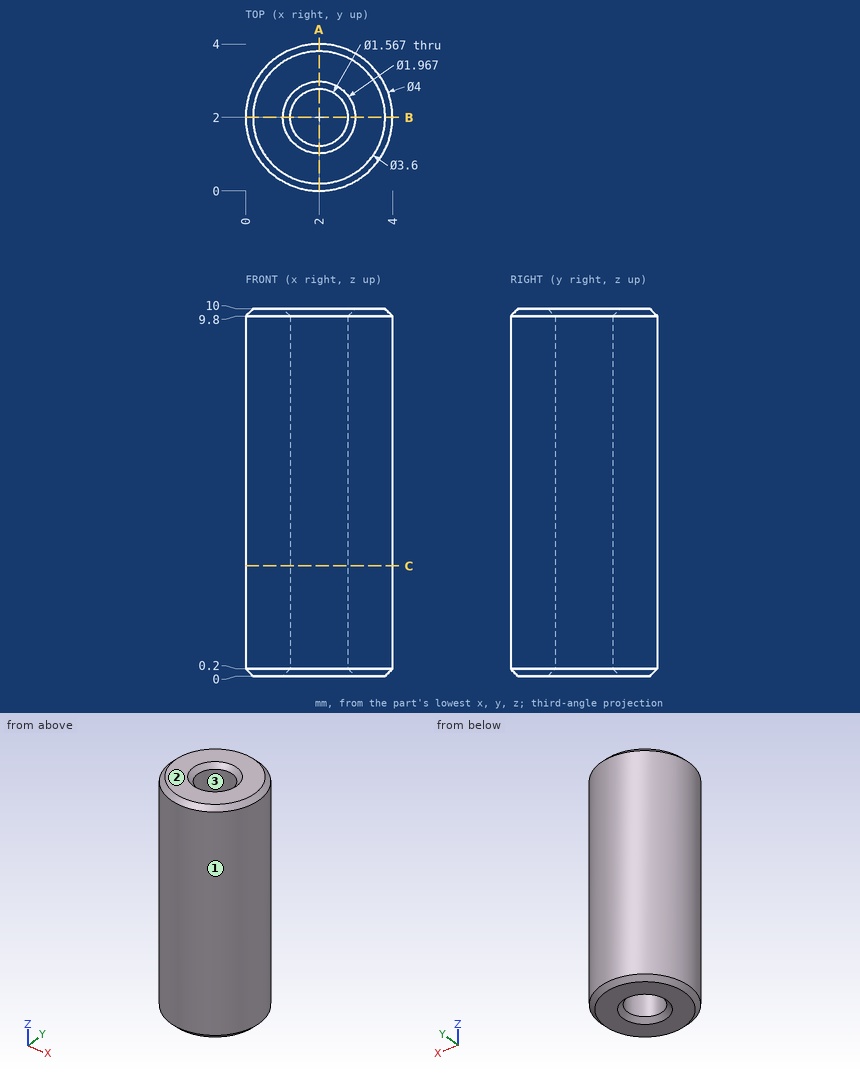
Check sheet for the drawn part. Datum: minimum x, y, z corner. Units: mm. Round coordinates to 2 decimals unless told otherwise and drop trailing zeros. Loops run counter-clockwise (first coordinate to the right, second up) from the corner with the lowest first, then second, coordinate; pieces in that order, holes last. Notation, with made-up numbers: (-36.5, -3.5) -> (8.5, -3.5) arc R11 ccw to (8.5, 0.5) -> close; hole circle Ø6 at (63.25, -30.5). An arc over 180 degrees is marked (long way). Put each result on its own line as item: value. Start each with the question number.
1. Section check C-C (z = 3). Enter the section's corners in (x, y).
2. Draft check along Y on the marked faces 1, 2 and 3. Enter one of: +Y half, -Y half, draft (parallel to the pull), parting line (faces both ways), or undercut.
3. Section check A-A (x = 2). Enter the section's corners in (y, z).
4. Gauge pin test, flat ends, axial feed: pin 1 (2 mm diameter, centred on x = 1, z = 2, fed in from -Y); pin 2 (1 mm diameter, centred on y = 1, z = 3, fed in from +X). Record the tip position at first contact, or that the pin passes through.
5. Scan lines: probe 1 along Y at (x, z) = (2, 7.5); probe 2 along X at (y, z) = (2.65, 2.5). Record each from-to range of solid material in increasing order.
Findings:
1. outline: circle Ø4 at (2, 2); hole circle Ø1.57 at (2, 2)
2. face 1: parting line
2. face 2: draft
2. face 3: undercut
3. outline: (0, 0.2) -> (0.2, 0) -> (1.02, 0) -> (1.22, 0.2) -> (1.22, 9.8) -> (1.02, 10) -> (0.2, 10) -> (0, 9.8) -> close; (2.78, 0.2) -> (2.98, 0) -> (3.8, 0) -> (4, 0.2) -> (4, 9.8) -> (3.8, 10) -> (2.98, 10) -> (2.78, 9.8) -> close
4. pin 1: stops at y = 0
4. pin 2: stops at x = 3.94
5. probe 1: y = 0 to 1.22, 2.78 to 4
5. probe 2: x = 0.11 to 1.56, 2.44 to 3.89
